Can you work these out from the model? Positions are in its coordinate system, mm. Face numbers are marked on the shaded views. A direction names the side the tool comes from. Round coordinates to 2 decimals unless told otherwise and drop trailing zeros. Write each loop counter-clockwise with the first axis right and the second up, starting at its lowest first coordinate (ties: lowest second). Pieces come first, ordered by that corner, then holes. Notation, with made-up numbers: (-12.75, 0) - (-6.75, 0) arc R25 cw to (-6.75, 14) - close; hole circle Ø6 at (-32.75, -8.75). An arc over 180 degrees is marked (long way). One line per item, written item: value. Start each with the question number.
(1) I want a section at A-A on y = 0.65. List the corners of the cut face in (x, z) for me, plus the area to 3 significant figures.
(2) Thinking about a two-plate mould opening in X: for the marked faces 3, 4 and 5, which applies, +X half, -X half, draft (parallel to the pull), parting line (faces both ways), or undercut?
(3) If I drill on L1, parallel to X at y = 3.5, z = 20; L2, parallel to Z at x = -17.5, y = 1.7; L3, parallel to Z at x = -10.5, y = 1.55, over which ranges is the centre line in solid material (lowest first)? Write a range as from..to.
(4) On a 3-axis mill with a long thin cutter (end or side, diameter ignored), from which of +Z, -Z, +X, -X, +Y, -Y can I reach the whole of each face in a straight line? I mean the marked faces 1 and 2. Say none if no direction works.
(5) I want a section at D-D on x = -5.5. List the corners of the cut face in (y, z) for me, plus the area to 3 significant figures.
(6) I'm going to push flat-ended pins straight in: pin 1 Ø2 at (x, z) = (-14, 7) entering from -Y; pin 2 Ø3 at (x, z) = (-15.5, 9) entering from +Y; pin 3 Ø1.6 at (x, y) = (-5, 0.5) entering from -Z; pin 4 Ø0.9 at (x, y) = (-4, 3) entering from -Z. Where does each tip first touch, or does it pass through?
(7) I want a section at B-B on x = 7.5. List the corners of the cut face in (y, z) for me, plus the area to 3 significant figures.
(8) I want a section at C-C on z = 19.5. List the corners of the cut face in (x, y) for me, plus the area to 3 significant figures.
Autodesk Fusion 360 part; units mm, degrees
sketch "Sketch3" plane through (0, 0, 0) normal (0, 1, 0) x (1, 0, 0)
  line L0 (11, 2.882) -> (-21, 2.882)
  line L1 (-21, 2.882) -> (-21, -32.118)
  line L2 (-21, -32.118) -> (11, -32.118)
  line L3 (11, -32.118) -> (11, 2.882)
  line L4 (-5, -24.618) -> (-5, 2.882)
  circle A0 centre (-17.5, -24.618) radius 1.5
  circle A1 centre (7.5, -24.618) radius 1.5
  line L5 (-17.5, -24.618) -> (7.5, -24.618)
  line L6 (-5, 0.0503) -> (-18, 0.0503)
  line L7 (-5, 0.0503) -> (8, 0.0503)
  line L8 (-18, 0.0503) -> (-18, -23.2038)
  line L9 (8, 0.0503) -> (8, -23.2038)
  line L10 (-5, 2.882) -> (-13, 2.882)
  line L11 (-5, 2.882) -> (3, 2.882)
  line L12 (-13, 2.882) -> (-13, -9.118)
  line L13 (3, 2.882) -> (3, -9.118)
  line L14 (-13, -9.118) -> (3, -9.118)
  dimension "d32" = 35
  dimension "d33" = 32
  dimension "d58" = 27.5
  dimension "d61" = 3
  dimension "d62" = 3
  dimension "d63" = 13
  dimension "d64" = 13
  dimension "d66" = 8
  dimension "d67" = 8
  dimension "d68" = 12
  dimension "d69" = 12
  dimension "d70" = 16
  dimension "d71" = 23.2541
extrude "Extrude7" add sketch "Sketch3" along normal blind 4.5 contours L0 L1 L2 L3 A0 A1 L5 L6 L7 L8 L9 L12 L13
extrude "Extrude8" add sketch "Sketch3" along normal blind 1.5 contours L4 A1 L5 L7 L9 L13 L14 | L4 A0 L5 L6 L8 L12 L14
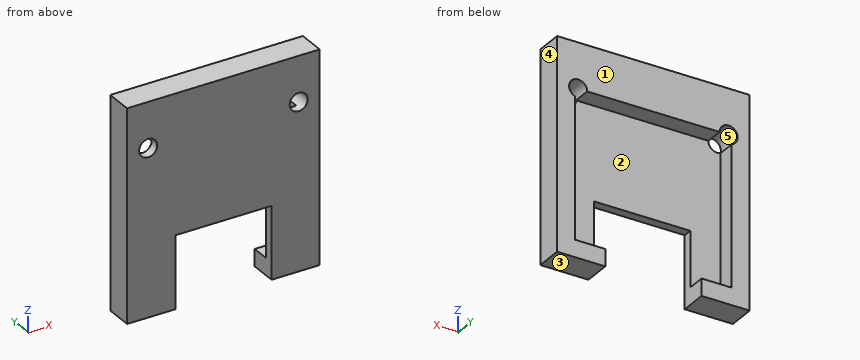
Established:
1. outline: (-21, -2.88) - (-13, -2.88) - (-13, 9.12) - (3, 9.12) - (3, -2.88) - (11, -2.88) - (11, 32.12) - (-21, 32.12) - close; hole circle Ø3 at (-17.5, 24.62); hole circle Ø3 at (7.5, 24.62)
1. area: 914 mm2
2. face 3: draft
2. face 4: +X half
2. face 5: undercut
3. L1: -21..-18, 8..11
3. L2: -2.88..-0.05, 26.12..32.12
3. L3: 24.62..32.12
4. face 1: +Z, -Z, +X, -X, +Y
4. face 2: +Y
5. outline: (0, 9.12) - (1.5, 9.12) - (1.5, 24.62) - (4.5, 24.62) - (4.5, 32.12) - (0, 32.12) - close
5. area: 57.0 mm2
6. pin 1: y = 0
6. pin 2: y = 1.5
6. pin 3: z = 9.12
6. pin 4: z = 24.62
7. outline: (0, -2.88) - (4.5, -2.88) - (4.5, -0.05) - (1.5, -0.05) - (1.5, 23.12) - (0, 23.12) - close; (0, 26.12) - (4.5, 26.12) - (4.5, 32.12) - (0, 32.12) - close
7. area: 74.5 mm2
8. outline: (-21, 0) - (11, 0) - (11, 4.5) - (8, 4.5) - (8, 1.5) - (-18, 1.5) - (-18, 4.5) - (-21, 4.5) - close
8. area: 66.0 mm2
